For this review, take the finished solid that the model builds, in its own axes (mm). Face numbers are marked on the shaded views. A direction names the side the tool comes from. Round coordinates to 2 decimals unless told otherwise and drop trailing zeros. Write each loop counter-clockwise with the first axis right and the second up, starting at its lowest first coordinate (ties: lowest second). Pieces come first, ordered by that corner, then holes. Notation, with made-up numbers: (17.5, 38.25) -> (23.5, 38.25) arc R20 cw to (23.5, 46.25) -> close; hole circle Ø9 at (86.25, 22). An arc over 180 degrees is marked (long way). Write each question's results on one line, items separated by ' | '. Start each with the question number.
Item 1: Add section D-D (z = -6.25). State the section outline as (x, y) points.
Item 2: Clearance check with flat-ended pins moving along their axes: pin 1 (4 mm diameter, centred on x = -4, y = -9.5, fed in from -Z); pin 2 (1 mm diameter, centred on y = -59, z = -6, fed in from -X); pin 3 (1.5 mm diameter, centred on y = -43, z = -3.5, fed in from -X). State where each tip first meets the part, or that it passes through.
Item 3: Tool access review of the marked faces 4 and 5: name each direction out of +Z, -Z, +X, -X, +Y, -Y from which nothing blocks a thin tool from reaching the whole face with its end or side.
Item 4: To check wall thickness, follow line 1 along Z through (x, y) = (0, -65.45); line 2 along X through (y, z) = (-43, -0.5); line 3 along Y through (x, z) = (2.75, -4). State the ranges of each line that lie inside material, in increasing order.
Item 5: Add section A-A (z = 0). State the section outline as (x, y) points, plus the area to 3 significant figures.
Item 6: The part is to be moulded in two halves that separate along X. For the marked faces 1, 2 and 3, say which applies: +X half, -X half, draft (parallel to the pull), parting line (faces both ways), or undercut.
Item 7: Add section B-B (x = 0). State the section outline as (y, z) points, plus the area to 3 significant figures.
Item 8: Add section C-C (y = -33). State the section outline as (x, z) points, plus the area to 3 significant figures.
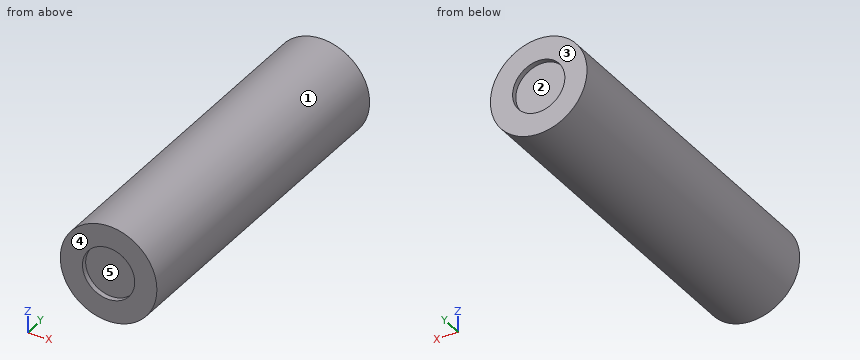
from build123d import *

# Parameters (mm, degrees)
F0_R     = 9.25
F1_DEPTH = 66
F2_R     = 5
F3_DEPTH = 1
F4_R     = 5
F5_DEPTH = 1


with BuildPart() as f1:
    # F0 (on Front) → F1 (new body)
    with BuildSketch(Plane.XZ):
        Circle(F0_R)
    extrude(amount=F1_DEPTH)

    # F2 (on Front) → F3 (cut)
    with BuildSketch(Plane.XZ):
        Circle(F2_R)
    extrude(amount=F3_DEPTH, mode=Mode.SUBTRACT)

    # F4 (on face) → F5 (cut)
    with BuildSketch(Plane.XZ.offset(66)):
        Circle(F4_R)
    extrude(amount=-F5_DEPTH, mode=Mode.SUBTRACT)


solid = f1.part
Responses:
1) outline: (-6.82, -66) -> (6.82, -66) -> (6.82, 0) -> (-6.82, 0) -> close
2) pin 1: stops at z = -9.03 | pin 2: stops at x = -7.44 | pin 3: stops at x = -8.83
3) face 4: +Z, -Z, +X, -X, -Y | face 5: -Y
4) line 1: z = -9.25 to -5, 5 to 9.25 | line 2: x = -9.24 to 9.24 | line 3: y = -65 to -1
5) outline: (-9.25, -66) -> (-5, -66) -> (-5, -65) -> (5, -65) -> (5, -66) -> (9.25, -66) -> (9.25, 0) -> (5, 0) -> (5, -1) -> (-5, -1) -> (-5, 0) -> (-9.25, 0) -> close | area: 1,200 mm^2
6) face 1: parting line | face 2: undercut | face 3: draft
7) outline: (-66, -9.25) -> (0, -9.25) -> (0, -5) -> (-1, -5) -> (-1, 5) -> (0, 5) -> (0, 9.25) -> (-66, 9.25) -> (-66, 5) -> (-65, 5) -> (-65, -5) -> (-66, -5) -> close | area: 1,200 mm^2
8) outline: circle Ø18.5 at (0, 0) | area: 269 mm^2
